```python
from build123d import *

# Parameters (mm, degrees)
SKETCH_1_W          = 62
SKETCH_1_H          = 26
EXTRUDE_1_DEPTH     = 4
SKETCH_2_R          = 1.5
CUT_EXTRUDE_1_DEPTH = 68.349832962
SKETCH_3_W          = 50
SKETCH_3_H          = 5
EXTRUDE_2_DEPTH     = 9
SKETCH_4_R          = 4.5
EXTRUDE_3_DEPTH     = 13
SKETCH_5_W          = 8
SKETCH_5_H          = 7
EXTRUDE_4_DEPTH     = 9
SKETCH_6_W          = 9
SKETCH_6_H          = 16
EXTRUDE_5_DEPTH     = 5


with BuildPart() as part:
    # 草图1 → 凸台-拉伸1 (new body)
    with BuildSketch(Plane(origin=(0, 0, 0), x_dir=(1, 0, 0), z_dir=(0, 1, 0))):
        with Locations((31, 13)):
            Rectangle(SKETCH_1_W, SKETCH_1_H)
    extrude(amount=EXTRUDE_1_DEPTH)

    # 草图2 → 切除-拉伸1 (cut, through all)
    with BuildSketch(Plane(origin=(0, 4, 0), x_dir=(1, 0, 0), z_dir=(0, 1, 0))):
        with Locations(Location((3, 23, 0), (0, 0, 270))):
            Circle(SKETCH_2_R)
        with Locations(Location((3, 3, 0), (0, 0, 270))):
            Circle(SKETCH_2_R)
        with Locations(Location((59, 3, 0), (0, 0, 270))):
            Circle(SKETCH_2_R)
        with Locations(Location((59, 23, 0), (0, 0, 270))):
            Circle(SKETCH_2_R)
    extrude(amount=-CUT_EXTRUDE_1_DEPTH, mode=Mode.SUBTRACT)

    # 草图3 → 凸台-拉伸2 (add)
    with BuildSketch(Plane(origin=(0, 4, 0), x_dir=(1, 0, 0), z_dir=(0, 1, 0))):
        with Locations((31, 3)):
            Rectangle(SKETCH_3_W, SKETCH_3_H)
    extrude(amount=EXTRUDE_2_DEPTH)

    # 草图4 → 凸台-拉伸3 (add)
    with BuildSketch(Plane(origin=(0, 4, 0), x_dir=(1, 0, 0), z_dir=(0, 1, 0))):
        with Locations(Location((18, 21.5, 0), (0, 0, 90))):
            Circle(SKETCH_4_R)
    extrude(amount=EXTRUDE_3_DEPTH)

    # 草图5 → 凸台-拉伸4 (add)
    with BuildSketch(Plane(origin=(0, 4, 0), x_dir=(1, 0, 0), z_dir=(0, 1, 0))):
        with Locations((32, 22)):
            Rectangle(SKETCH_5_W, SKETCH_5_H)
    extrude(amount=EXTRUDE_4_DEPTH)

    # 草图6 → 凸台-拉伸5 (add)
    with BuildSketch(Plane(origin=(0, 4, 0), x_dir=(1, 0, 0), z_dir=(0, 1, 0))):
        with Locations((-1.5, 13)):
            Rectangle(SKETCH_6_W, SKETCH_6_H)
    extrude(amount=EXTRUDE_5_DEPTH)


solid = part.part
```
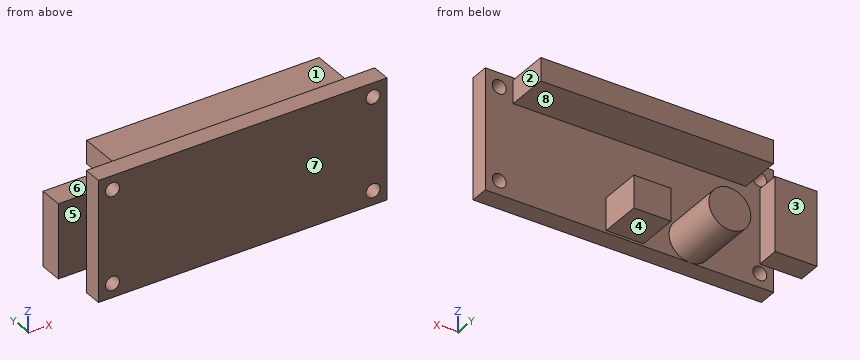
Build history of the part. All positions in model axes, mm. Face numbers are marked on the shaded views. A direction names the side the tool comes from. Round coordinates to 2 decimals unless told otherwise and drop trailing zeros. Order: outer loops, then holes, each group sorted by start corner. A loop starts at its lowest first (then second) coordinate and runs counter-clockwise, first axis right, second up. Notation, with made-up numbers: (84, -18.75) -> (142, -18.75) arc R18 ccw to (142, 13.25) -> close; hole circle Ø8 at (56, 46.25). An arc over 180 degrees is marked (long way). Answer in a Markdown table with one row per item.
1) Band-saw the part on A-A on x = 59. Give the cut face in (y, z), and give its area (3 significant figures).
Values:
| item | result |
|---|---|
| outline | (0, -26) -> (4, -26) -> (4, -24.5) -> (0, -24.5) -> close; (0, -21.5) -> (4, -21.5) -> (4, -4.5) -> (0, -4.5) -> close; (0, -1.5) -> (4, -1.5) -> (4, 0) -> (0, 0) -> close |
| area | 80.0 mm2 |
2) Band-saw the part on D-D on y = 10.5. Give the cut face in (x, z).
Values:
| item | result |
|---|---|
| outline | (6, -5.5) -> (56, -5.5) -> (56, -0.5) -> (6, -0.5) -> close; circle Ø9 at (18, -21.5); (28, -25.5) -> (36, -25.5) -> (36, -18.5) -> (28, -18.5) -> close |
3) Mould opens along Z. For the marked faces 6, 7 and 8 say: released by +Z, released by -Z, zero draft, split by the parting line, or undercut.
Values:
| item | result |
|---|---|
| face 6 | released by +Z |
| face 7 | zero draft |
| face 8 | undercut |
4) Band-saw the part on B-B on y = 7.75. Give the cut face in (x, z), and give its area (3 significant figures).
Values:
| item | result |
|---|---|
| outline | (-6, -21) -> (3, -21) -> (3, -5) -> (-6, -5) -> close; (6, -5.5) -> (56, -5.5) -> (56, -0.5) -> (6, -0.5) -> close; circle Ø9 at (18, -21.5); (28, -25.5) -> (36, -25.5) -> (36, -18.5) -> (28, -18.5) -> close |
| area | 514 mm2 |
5) Wall check: L1, parallel to X at y = 1.95, z = -23; L2, parallel to X at y = 7.75, z = -5.25; L3, parallel to X at y = 1.75, z = -1.75. Give the ranges that are in metal, low to high.
Values:
| item | result |
|---|---|
| L1 | 0 to 1.5, 4.5 to 57.5, 60.5 to 62 |
| L2 | -6 to 3, 6 to 56 |
| L3 | 0 to 2.17, 3.83 to 58.17, 59.83 to 62 |
6) Band-saw the part on C-C on z = -3. Give the cut face in (x, y), and give its area (3 significant figures).
Values:
| item | result |
|---|---|
| outline | (0, 0) -> (1.5, 0) -> (1.5, 4) -> (0, 4) -> close; (4.5, 0) -> (57.5, 0) -> (57.5, 4) -> (56, 4) -> (56, 13) -> (6, 13) -> (6, 4) -> (4.5, 4) -> close; (60.5, 0) -> (62, 0) -> (62, 4) -> (60.5, 4) -> close |
| area | 674 mm2 |
7) Which spindle directions (+Z, -Z, +X, -X, +Y, -Y) get a long thin tool onto all of the face, cutting with end or side? Do the marked faces 1, 2, 3, 4 and 5. Say none if no direction does.
Values:
| item | result |
|---|---|
| face 1 | +Z, +X, -X, +Y |
| face 2 | +Z, -Z, +X, +Y |
| face 3 | +Z, -Z, -X, +Y |
| face 4 | -Z, +X, +Y |
| face 5 | +Z, -Z, -X, -Y |
8) Pin check, flat tips, straight feed: P1, Ø2.5, axis at x = 36, y = 8.5, coming from the +Z side; P2, Ø4, axis at x = -1.5, y = 6.5, coming from the -Z side; P3, Ø1.8, axis at x = -3, z = -11.5, coming from the -Y side; P4, Ø2.5, axis at x = 3, z = -23, coming from the -Y side. Stop position of each tip, or through.
Values:
| item | result |
|---|---|
| P1 | z = -0.5 |
| P2 | z = -21 |
| P3 | y = 4 |
| P4 | through |
